from build123d import *

# Parameters (mm, degrees)
SKETCH2_W           = 6
SKETCH2_H           = 18
BOSS_EXTRUDE1_DEPTH = 18
SKETCH3_R           = 2.25
CUT_EXTRUDE1_DEPTH  = 21.346989949
SKETCH4_W           = 4.5
SKETCH4_H           = 12
CUT_EXTRUDE2_DEPTH  = 3
SKETCH5_R           = 1.05
CUT_EXTRUDE3_DEPTH  = 21.346989949
SKETCH8_W           = 4.5
SKETCH8_H           = 7
CUT_EXTRUDE6_DEPTH  = 10


with BuildPart() as part:
    # Sketch2 → Boss-Extrude1 (new body)
    with BuildSketch(Plane.XY):
        Rectangle(SKETCH2_W, SKETCH2_H)
    extrude(amount=BOSS_EXTRUDE1_DEPTH)

    # Sketch3 → Cut-Extrude1 (cut, through all)
    with BuildSketch(Plane.XY.offset(18)):
        with Locations((0, -6)):
            Circle(SKETCH3_R)
    extrude(amount=-CUT_EXTRUDE1_DEPTH, mode=Mode.SUBTRACT)

    # Sketch4 → Cut-Extrude2 (cut)
    with BuildSketch(Plane(origin=(3, 0, 0), x_dir=(0, 0, -1), z_dir=(1, 0, 0))):
        with Locations((-9, 3)):
            Rectangle(SKETCH4_W, SKETCH4_H)
    extrude(amount=-CUT_EXTRUDE2_DEPTH, mode=Mode.SUBTRACT)

    # Sketch5 → Cut-Extrude3 (cut, through all)
    with BuildSketch(Plane.XY.offset(18)):
        with Locations((0, 4)):
            Circle(SKETCH5_R)
    extrude(amount=-CUT_EXTRUDE3_DEPTH, mode=Mode.SUBTRACT)

    # Sketch8 → Cut-Extrude6 (cut)
    with BuildSketch(Plane(origin=(3, 0, 0), x_dir=(0, 0, -1), z_dir=(1, 0, 0))):
        with Locations((-9, 5.5)):
            Rectangle(SKETCH8_W, SKETCH8_H)
    extrude(amount=-CUT_EXTRUDE6_DEPTH, mode=Mode.SUBTRACT)


solid = part.part
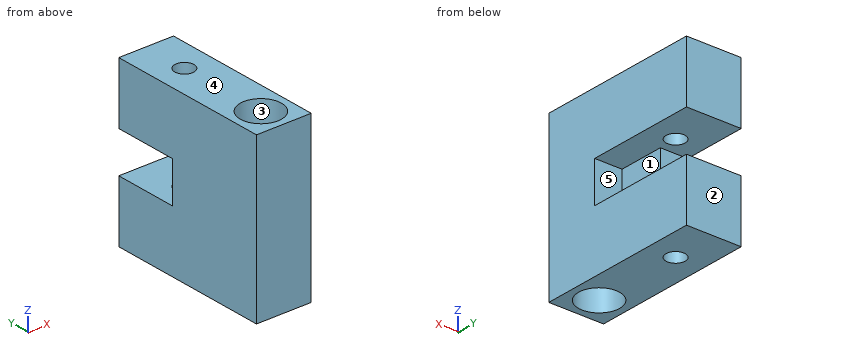
Geometry: final body of the model. Coordinates: model frame, mm. Face numbers are marked on the shaded views. A direction names the side the tool comes from. Give positions to 0.01 mm unless a question says otherwise; leave off trailing zeros. Write each loop counter-clockwise with the first axis right and the second up, starting at its lowest first coordinate (ties: lowest second). Pieces come first, ordered by that corner, then holes. Notation, with made-up numbers: (69.25, -24.75) -> (123.25, -24.75) arc R19 cw to (123.25, 8.25) -> close; hole circle Ø9 at (-5.5, -8.75). An arc over 180 degrees is marked (long way). Answer in a Markdown table with one row per item.
(1) Section query D-D on x = -2. Return loops of the section in (y, z).
Answers below:
| item | result |
|---|---|
| outline | (-9, 0) -> (-7.03, 0) -> (-7.03, 18) -> (-9, 18) -> close; (-4.97, 0) -> (9, 0) -> (9, 6.75) -> (2, 6.75) -> (2, 11.25) -> (9, 11.25) -> (9, 18) -> (-4.97, 18) -> close |
(2) Section query B-B on z = 8.25. Return loops of the section in (x, y).
Answers below:
| item | result |
|---|---|
| outline | (-3, -9) -> (3, -9) -> (3, -3) -> (0, -3) -> (0, 2) -> (-3, 2) -> close; hole circle Ø4.5 at (0, -6) |
(3) Set-up query: the marked faces 1 and 2. Return all of +Z, -Z, +X, -X, +Y, -Y with unobstructed straight access to the full face (end or side cutting, diameter ignored); none if empty.
Answers below:
| item | result |
|---|---|
| face 1 | +X, +Y |
| face 2 | +Z, -Z, +X, -X, +Y |
(4) Section query A-A on y = 5.5. Return loops of the section in (x, z), then the cut area to 3 significant figures.
Answers below:
| item | result |
|---|---|
| outline | (-3, 0) -> (3, 0) -> (3, 6.75) -> (-3, 6.75) -> close; (-3, 11.25) -> (3, 11.25) -> (3, 18) -> (-3, 18) -> close |
| area | 81.0 mm^2 |
(5) Section query C-C on x = 0.35. Return loops of the section in (y, z), then the cut area to 3 significant figures.
Answers below:
| item | result |
|---|---|
| outline | (-9, 0) -> (-8.22, 0) -> (-8.22, 18) -> (-9, 18) -> close; (-3.78, 0) -> (3.01, 0) -> (3.01, 6.75) -> (-3, 6.75) -> (-3, 11.25) -> (3.01, 11.25) -> (3.01, 18) -> (-3.78, 18) -> close; (4.99, 0) -> (9, 0) -> (9, 6.75) -> (4.99, 6.75) -> close; (4.99, 11.25) -> (9, 11.25) -> (9, 18) -> (4.99, 18) -> close |
| area | 163 mm^2 |
(6) Pin query (flat end, axial travel): pin 1 (3.5 mm diameter, centred on x = -1.5, z = 9, fed in from +Y); pin 2 (1.5 mm diameter, centred on x = 1, z = 9, fed in from +Y). Return the tip coordinate at first contact, or that it passes through.
Answers below:
| item | result |
|---|---|
| pin 1 | y = 2 |
| pin 2 | y = -3 |
(7) Draft query along Z for the marked faces 3, 4 and 5. Return one class per face: +Z half, -Z half, draft (parallel to the pull), parting line (faces both ways), or undercut.
Answers below:
| item | result |
|---|---|
| face 3 | draft |
| face 4 | +Z half |
| face 5 | undercut |
(8) Ray query, line 1 along Y through (x, z) = (0, 12); line 2 along Z through (x, y) = (-2.2, 6.75); line 3 along Y through (x, z) = (0.9, 14.75). Return the intervals inside material, ascending. Write a range as [from, to].
Answers below:
| item | result |
|---|---|
| line 1 | [-9, -8.25], [-3.75, 2.95], [5.05, 9] |
| line 2 | [0, 6.75], [11.25, 18] |
| line 3 | [-9, -8.06], [-3.94, 3.46], [4.54, 9] |
